Design review of the part built by this model. Coordinates are the model's own, in mm. A direction names the side the tool comes from. Round coordinates to 2 decimals unless told otherwise and drop trailing zeros. Loops run counter-clockwise (first coordinate to the right, second up) from the corner with the lowest first, then second, coordinate; pieces in that order, holes last. Notation, with made-up numbers: (-39.75, 60.5) - (2.25, 60.5) arc R13 ccw to (2.25, 80.5) - close; hole circle Ø9 at (4.25, 25.5). An arc over 180 degrees is marked (long way). Answer as CSV lines item,"result". Start each with the question number.
(1) Consider section B-B (y = -50). Give the boundary of the cut face in (x, z).
(2) Consider section A-A (x = -12.5). Give the boundary of the cut face in (y, z).
(3) For faces 4 (the flat face through (-8.75, -22, -4)), 5 (the flat face through (9, -106, -4)), 6 (the flat face through (-21, -100, -4)), 7 (the flat face through (21, -100, -4)), list the 3-axis set-ups (+Z, -Z, +X, -X, +Y, -Y) from which the entire face can be reached by the end or side of a thin tool; tool diameter is ignored.
(4) Mouldability with a two-part tool opening along X and no side actions: class faces 1 (the cylindrical face through (0.495, 22.495, -3.944)), 2 (the flat face through (13, -108, -4)), 3 (the flat face through (13, -84, -1)) as released by +X, released by -X, zero draft, split by the parting line, or undercut.
(5) Consider section C-C (x = 7). Give the boundary of the cut face in (y, z).
(6) Consider section D-D (x = 12). Give the boundary of the cut face in (y, z).
(7) Wall thickness on L1, parallel to Y at x = 0, z = -4.25; L2, parallel to Y at x = 0, z = -3.75; L3, parallel to Y at x = 3, z = -3: over which ranges is each line inside the solid? List them lowest first.
(8) For P1, Ø1, axis at y = -29, z = -1, coming from the -X side; P2, Ø2, axis at x = 7.5, z = -5, coming from the -Y side; P3, Ø4.5, axis at y = -43.5, z = -2.5, coming from the +X side; P4, Ø2.5, axis at y = -104, z = -4, coming from the -X side, all flat-tipped, find the tip position at first contact; note any pin that passes through.
from build123d import *

# Parameters (mm, degrees)
ARM_BOSS_EXTRUDE1_DEPTH                    = 8
STEPPER_CUT_EXTRUDE1_DEPTH                 = 8
CABLE_CUT_EXTRUDE2_DEPTH                   = 1
ULN2003_MODULE_CUT_EXTRUDE3_DEPTH          = 4
SKETCH6_W                                  = 8
SKETCH6_H                                  = 8
PUZZLE_SLOT_BOSS_EXTRUDE2_DEPTH            = 8
SKETCH7_R                                  = 1.75
MOUNTING_HOLES_CUT_EXTRUDE4_DEPTH          = 8
PUZZLE_SLOT_SCREW_HOLES_CUT_EXTRUDE5_REACH = 118.155
SKETCH8_R                                  = 1.5
SKETCH10_W                                 = 4
SKETCH10_H                                 = 3.063353071
CABLE_OUTPUT_CUT_EXTRUDE6_DEPTH            = 1
SIDE_PUZZLE_SLOT_CUT_EXTRUDE7_DEPTH        = 8
CABLE_LOWER_CUT_EXTRUDE8_DEPTH             = 1


with BuildPart() as part:
    # Sketch2 → Arm Boss-Extrude1 (new body)
    with BuildSketch(Plane.XY):
        with BuildLine():
            Line((-22.5, 0), (-25, -100))
            Line((-25, -100), (0, -100))
            Line((0, -100), (25, -100))
            Line((25, -100), (22.5, 0))
            ThreePointArc((22.5, 0), (0, 22.5), (-22.5, 0))
        make_face()
    extrude(amount=-ARM_BOSS_EXTRUDE1_DEPTH)

    # Sketch3 → Stepper Cut-Extrude1 (cut)
    with BuildSketch(Plane.XY):
        with BuildLine():
            Line((-8.75, -18.928746497), (-8.75, -25.928746497))
            Line((-8.75, -25.928746497), (0, -25.928746497))
            Line((0, -25.928746497), (8.75, -25.928746497))
            Line((8.75, -25.928746497), (8.75, -18.928746497))
            ThreePointArc((8.75, -18.928746497), (0, 6), (-8.75, -18.928746497))
        make_face()
    extrude(amount=-STEPPER_CUT_EXTRUDE1_DEPTH, mode=Mode.SUBTRACT)

    # Sketch4 → Cable Cut-Extrude2 (cut)
    with BuildSketch(Plane.XY):
        Polygon((-2, -25.928746497), (2, -25.928746497), (2, -30.928746497), (0, -30.928746497), (-2, -30.928746497), align=None)
    extrude(amount=-CABLE_CUT_EXTRUDE2_DEPTH, mode=Mode.SUBTRACT)

    # Sketch5 → ULN2003 Module Cut-Extrude3 (cut)
    with BuildSketch(Plane.XY):
        Polygon((-16, -30.928746497), (16, -30.928746497), (16, -67.928746497), (0, -67.928746497), (-16, -67.928746497), align=None)
    extrude(amount=-ULN2003_MODULE_CUT_EXTRUDE3_DEPTH, mode=Mode.SUBTRACT)

    # Sketch6 → Puzzle Slot Boss-Extrude2 (add)
    with BuildSketch(Plane.XZ.offset(100)):
        with Locations((-13, -4)):
            Rectangle(SKETCH6_W, SKETCH6_H)
        with Locations((13, -4)):
            Rectangle(SKETCH6_W, SKETCH6_H)
    extrude(amount=PUZZLE_SLOT_BOSS_EXTRUDE2_DEPTH)

    # Sketch7 → Mounting Holes Cut-Extrude4 (cut)
    with BuildSketch(Plane.XY):
        with Locations((-18.45, -9.75)):
            Circle(SKETCH7_R)
        with Locations((18.45, -9.75)):
            Circle(SKETCH7_R)
    extrude(amount=-MOUNTING_HOLES_CUT_EXTRUDE4_DEPTH, mode=Mode.SUBTRACT)

    # Puzzle Slot Screw Holes Cut-Extrude5: up to this face of the body (flat: up to its plane)
    puzzle_slot_screw_holes_cut_extrude5_end = Plane(part.part.faces().sort_by_distance((17, -104, -4))[0])
    # Sketch8 → Puzzle Slot Screw Holes Cut-Extrude5 (cut, up to the picked face)
    with BuildSketch(Plane.ZY.offset(17), mode=Mode.PRIVATE) as puzzle_slot_screw_holes_cut_extrude5_sk1:
        with Locations(Location((-4, -104, 0), (0, 0, 270))):
            Circle(SKETCH8_R)
    puzzle_slot_screw_holes_cut_extrude5_tool1 = split(extrude(puzzle_slot_screw_holes_cut_extrude5_sk1.sketch, amount=-PUZZLE_SLOT_SCREW_HOLES_CUT_EXTRUDE5_REACH, mode=Mode.PRIVATE), bisect_by=puzzle_slot_screw_holes_cut_extrude5_end, keep=Keep.BOTH, mode=Mode.PRIVATE)
    add(puzzle_slot_screw_holes_cut_extrude5_tool1.solids().sort_by(Axis((-17, -104, -4), (1, 0, 0)))[0], mode=Mode.SUBTRACT)

    # Sketch10 → Cable Output Cut-Extrude6 (cut)
    with BuildSketch(Plane.XY.offset(-1)):
        with Locations((0, -27.460423033)):
            Rectangle(SKETCH10_W, SKETCH10_H)
    extrude(amount=-CABLE_OUTPUT_CUT_EXTRUDE6_DEPTH, mode=Mode.SUBTRACT)

    # Sketch11 → Side Puzzle Slot Cut-Extrude7 (cut)
    with BuildSketch(Plane.XY):
        Polygon((-4, -86), (4, -86), (4, -78), (0, -78), (-4, -78), align=None)
    extrude(amount=-SIDE_PUZZLE_SLOT_CUT_EXTRUDE7_DEPTH, mode=Mode.SUBTRACT)

    # Sketch12 → Cable Lower Cut-Extrude8 (cut)
    with BuildSketch(Plane.XY):
        Polygon((15, -67.928746497), (10, -67.928746497), (10, -82.103104923), (10.5, -88.003309516), (10.5, -100), (15.5, -100), (15.5, -88.003309516), (15, -82.103104923), align=None)
    extrude(amount=-CABLE_LOWER_CUT_EXTRUDE8_DEPTH, mode=Mode.SUBTRACT)


solid = part.part
Determined:
1,outline,"(-23.75, -8) - (23.75, -8) - (23.75, 0) - (16, 0) - (16, -4) - (-16, -4) - (-16, 0) - (-23.75, 0) - close"
2,outline,"(-108, -8) - (-14.3, -8) - (-14.3, 0) - (-30.93, 0) - (-30.93, -4) - (-67.93, -4) - (-67.93, 0) - (-108, 0) - close; (-1.7, -8) - (18.71, -8) - (18.71, 0) - (-1.7, 0) - close; hole circle Ø3 at (-104, -4)"
3,face 4,"+Z, -Z"
3,face 5,"+Z, -Z, -Y"
3,face 6,"+Z, -Z, -X, -Y"
3,face 7,"+Z, -Z, +X, -Y"
4,face 1,"split by the parting line"
4,face 2,"zero draft"
4,face 3,"undercut"
5,outline,"(-100, -8) - (-25.93, -8) - (-25.93, 0) - (-30.93, 0) - (-30.93, -4) - (-67.93, -4) - (-67.93, 0) - (-100, 0) - close; (4.12, -8) - (21.38, -8) - (21.38, 0) - (4.12, 0) - close"
6,outline,"(-108, -8) - (-15.21, -8) - (-15.21, 0) - (-30.93, 0) - (-30.93, -4) - (-67.93, -4) - (-67.93, -1) - (-100, -1) - (-100, 0) - (-108, 0) - close; (-0.79, -8) - (19.03, -8) - (19.03, 0) - (-0.79, 0) - close; hole circle Ø3 at (-104, -4)"
7,L1,"y = -100 to -86, -78 to -25.93, 6 to 22.5"
7,L2,"y = -100 to -86, -78 to -67.93, -30.93 to -25.93, 6 to 22.5"
7,L3,"y = -100 to -86, -78 to -67.93, -30.93 to -25.93, 5.67 to 22.3"
8,P1,"stops at x = -23.24"
8,P2,"stops at y = -100"
8,P3,"stops at x = 23.64"
8,P4,"passes through"
